```python
from build123d import *

# Parameters (mm, degrees)
F0_R      = 4.175
F1_DEPTH  = 16
F2_R      = 4.125
F3_DEPTH  = 40
F4_R      = 4.125
F5_DEPTH  = 40
F6_R      = 3.85
F6_R_2    = 1.75
F7_DEPTH  = 8
F8_DEPTH  = 7
F6_R_3    = 5
F9_DEPTH  = 0.4
F10_R     = 1
F11_DEPTH = 10
F12_W     = 24
F12_H     = 16
F12_R     = 1
F13_DEPTH = 2


with BuildPart() as f1:
    # F0 (on Top) → F1 (new body)
    with BuildSketch(Plane.XY):
        Polygon((-42.5, 14.9807621135), (-56.3564064606, 6.9807621135), (-41.3564064606, -19), (-27.5, -11), (27.5, -11), (41.3564064606, -19), (56.3564064606, 6.9807621135), (42.5, 14.9807621135), (40.2017059222, 11), (0, 11), (-40.2017059222, 11), align=None)
        with Locations((-27.5, 0)):
            Circle(F0_R, mode=Mode.SUBTRACT)
        Circle(F0_R, mode=Mode.SUBTRACT)
        with Locations((27.5, 0)):
            Circle(F0_R, mode=Mode.SUBTRACT)
    extrude(amount=F1_DEPTH)

    # F2 (on face) → F3 (cut)
    with BuildSketch(Plane(origin=(17.1118602792, 29.6386114156, 0), x_dir=(-0.8660254038, 0.5, 0), z_dir=(0.5, 0.8660254038, 0))):
        with Locations((-37.3156986041, 8)):
            Circle(F2_R)
    extrude(amount=-F3_DEPTH, mode=Mode.SUBTRACT)

    # F4 (on face) → F5 (cut)
    with BuildSketch(Plane(origin=(-17.1118602792, 29.6386114156, 0), x_dir=(-0.8660254038, -0.5, 0), z_dir=(-0.5, 0.8660254038, 0))):
        with Locations((37.3156986041, 8)):
            Circle(F4_R)
    extrude(amount=-F5_DEPTH, mode=Mode.SUBTRACT)

    # F6 (on face) → F7 (join)
    with BuildSketch(Plane.XZ.offset(11)):
        with Locations((0, 8)):
            Circle(F6_R)
        with Locations((0, 8)):
            Circle(F6_R_2, mode=Mode.SUBTRACT)
    extrude(amount=F7_DEPTH)

    # F8 (cut): a face of the model
    f8_faces = [f1.faces().sort_by_distance(p)[0] for p in [
        (0, -11, 8),
    ]]
    extrude(f8_faces, amount=-F8_DEPTH, mode=Mode.SUBTRACT)

    # F6 (on face) → F9 (join)
    with BuildSketch(Plane.XZ.offset(11)):
        with Locations((0, 8)):
            Circle(F6_R_3)
        with Locations((0, 8)):
            Circle(F6_R, mode=Mode.SUBTRACT)
    extrude(amount=F9_DEPTH)

    # F10 (on face) → F11 (cut)
    with BuildSketch(Plane(origin=(0, 11, 0), x_dir=(-1, 0, 0), z_dir=(0, 1, 0))):
        with Locations((-4.75, 7.5)):
            Circle(F10_R)
        with Locations((4.75, 7.5)):
            Circle(F10_R)
    extrude(amount=-F11_DEPTH, mode=Mode.SUBTRACT)

    # F12 (on face) → F13 (cut)
    with BuildSketch(Plane(origin=(0, 11, 0), x_dir=(-1, 0, 0), z_dir=(0, 1, 0))):
        with Locations((0, 8)):
            Rectangle(F12_W, F12_H)
        with Locations((-4.75, 7.5)):
            Circle(F12_R, mode=Mode.SUBTRACT)
        with Locations((4.75, 7.5)):
            Circle(F12_R, mode=Mode.SUBTRACT)
    extrude(amount=-F13_DEPTH, mode=Mode.SUBTRACT)


solid = f1.part
```
Geometry check sheet. Reference: the model listing, model coordinates, mm. A direction names the side the tool comes from. Round coordinates to 2 decimals unless told otherwise and drop trailing zeros. Loops run counter-clockwise (first coordinate to the right, second up) from the corner with the lowest first, then second, coordinate; pieces in that order, holes last. Notation, with made-up numbers: (-23, 2.5) - (34, 2.5) arc R13 cw to (34, 14.5) - close; hole circle Ø3 at (10.5, 63). An arc over 180 degrees is marked (long way). Write item = value, one per line. Start each with the question number.
1. Depth check by flat-ended pin: pin 1 (1.5 mm diameter, centred on x = 36.5, z = 6, fed in from -Y); pin 2 (1.9 mm diameter, centred on x = 5, z = 7.5, fed in from +Y); pin 3 (0.6 mm diameter, centred on y = 10, z = 8.5, fed in from +X). Enter the tip coordinate at first touch or a pass-through.
2. Section check B-B on y = -14. Give the number of separate pieces and of enclosed holes in the cut face, then the cut area to 3 significant figures.
3. Set-up check for faces 1 (the face through (-0.651, -11.197, 12.957)), 2 (the face through (26, 11, 8)), 3 (the face through (31.252, -13.166, 4.332)): record each of +Z, -Z, +X, -X, +Y, -Y from which the full face is reachable in a straight line by a thin tool's end or side.
4. Thickness scan on line 1 (X direction, y = 4.5, z = 7.5); line 2 (X direction, y = 7.5, z = 7.5); line 3 (X direction, y = 8, z = 4.75). Record the ranges inside material, lowest first.
5. Section check A-A on x = 0. Enter the section's corners in (y, z) (3 decimals), then the cut area to 3 significant figures.
6. Mould release check, pull along X, two halves, no side actions. Record for faces 4 (the face through (-1, -6, 0)), 5 (the face through (41.37, 13.02, 7.89)), 6 (the face through (52.6, 9.15, 4.33)): released by +X, released by -X, zero draft, split by the parting line, or undercut.
Working result:
q1.pin_1 = -5.82
q1.pin_2 = 9
q1.pin_3 = 44.31
q2.separate_pieces = 3
q2.enclosed_holes = 1
q2.area = 308 mm^2
q3.face_1 = -Y
q3.face_2 = +Z, -Z, +Y
q3.face_3 = +Z, -Z, -Y
q4.line_1 = -54.92 to -50.41, -40.96 to -5.75, -3.75 to 3.75, 5.75 to 40.96, 50.41 to 54.92
q4.line_2 = -55.46 to -52.15, -42.69 to -5.75, -3.75 to 3.75, 5.75 to 42.69, 52.15 to 55.46
q4.line_3 = -54.59 to -50.64, -44.77 to 44.77, 50.64 to 54.59
q5.outline = (-19, 4.15) - (-11.4, 4.15) - (-11.4, 3) - (-11, 3) - (-11, 0) - (-4.175, 0) - (-4.175, 6.25) - (-19, 6.25) - close; (-19, 9.75) - (-4.175, 9.75) - (-4.175, 16) - (-11, 16) - (-11, 13) - (-11.4, 13) - (-11.4, 11.85) - (-19, 11.85) - close; (4.175, 0) - (9, 0) - (9, 16) - (4.175, 16) - close
q5.area = 197 mm^2
q6.face_4 = zero draft
q6.face_5 = undercut
q6.face_6 = released by +X
